The model under review builds one solid part; all positions refer to its coordinate system, in mm. Coordinates: 2 decimals unless noted, no trailing zeros. Order: outer loops, then holes, each group sorted by start corner. A loop starts at its lowest first (then second) coordinate and runs counter-clockwise, first axis right, second up. Notation, with made-up numbers: M 3.5,-2.75 L 18.5,-2.75 A13 ccw 18.5,14.25 Z; hole C 46,-30.75 d8. An arc over 180 degrees is marked long. Answer in a Markdown table with one row per item.
from build123d import *

# Parameters (mm, degrees)
BOSS_EXTRUDE1_DEPTH = 1
SKETCH2_R           = 2.55
CUT_EXTRUDE6_DEPTH  = 2.54
SKETCH3_R           = 1
CUT_EXTRUDE7_DEPTH  = 2.54


with BuildPart() as part:
    # Sketch1 → Boss-Extrude1 (new body)
    with BuildSketch(Plane(origin=(0, 0, 0), x_dir=(1, 0, 0), z_dir=(0, 1, 0))):
        with BuildLine():
            Line((-42.38, -50), (42.38, -50))
            ThreePointArc((42.38, -50), (47.768153673, -47.768153673), (50, -42.38))
            Line((50, -42.38), (50, 42.38))
            ThreePointArc((50, 42.38), (47.768153673, 47.768153673), (42.38, 50))
            Line((42.38, 50), (-42.38, 50))
            ThreePointArc((-42.38, 50), (-47.768153673, 47.768153673), (-50, 42.38))
            Line((-50, 42.38), (-50, -42.38))
            ThreePointArc((-50, -42.38), (-47.768153673, -47.768153673), (-42.38, -50))
        make_face()
    extrude(amount=BOSS_EXTRUDE1_DEPTH)

    # Sketch2 → Cut-Extrude6 (cut)
    with BuildSketch(Plane(origin=(0, 1, 0), x_dir=(1, 0, 0), z_dir=(0, 1, 0))):
        with Locations((0, 40)):
            Circle(SKETCH2_R)
        with Locations((40, 0)):
            Circle(SKETCH2_R)
        with Locations((0, -40)):
            Circle(SKETCH2_R)
        with Locations((-40, 0)):
            Circle(SKETCH2_R)
    extrude(amount=-CUT_EXTRUDE6_DEPTH, mode=Mode.SUBTRACT)

    # Sketch3 → Cut-Extrude7 (cut)
    with BuildSketch(Plane(origin=(0, 1, 0), x_dir=(1, 0, 0), z_dir=(0, 1, 0))):
        with Locations((0, 24)):
            Circle(SKETCH3_R)
        with Locations((24, 0)):
            Circle(SKETCH3_R)
        with Locations((0, -24)):
            Circle(SKETCH3_R)
        with Locations((-24, 0)):
            Circle(SKETCH3_R)
    extrude(amount=-CUT_EXTRUDE7_DEPTH, mode=Mode.SUBTRACT)


solid = part.part
(1) Take a section at B-B (x = -40). Write out the cut boundary in (y, z), then the cut area to 3 significant figures.
Report:
| item | result |
|---|---|
| outline | M 0,-50 L 1,-50 L 1,-2.55 L 0,-2.55 Z; M 0,2.55 L 1,2.55 L 1,50 L 0,50 Z |
| area | 94.9 mm^2 |
(2) Take a section at A-A (z = -40). Write out the cut boundary in (x, y).
Report:
| item | result |
|---|---|
| outline | M -50,0 L -2.55,0 L -2.55,1 L -50,1 Z; M 2.55,0 L 50,0 L 50,1 L 2.55,1 Z |
(3) The part is to be moulded in two halves that separate along X. For faces 1 (the flat face through (-1, 1, -1)), 2 (the cylindrical face through (-42.548, 0.507, -0.112)), 3 (the cylindrical face through (-47.709, 0.493, -47.827)), say which applies: +X half, -X half, draft (parallel to the pull), parting line (faces both ways), or undercut.
Report:
| item | result |
|---|---|
| face 1 | draft |
| face 2 | undercut |
| face 3 | -X half |
(4) To check wall thickness, follow line 1 (Z direction, x = 0, y = 0.2); line 2 (Z direction, x = -24, y = 0.45). State the ranges of each line that lie inside material, in increasing order. Write a range as [from, to].
Report:
| item | result |
|---|---|
| line 1 | [-50, -42.55], [-37.45, -25], [-23, 23], [25, 37.45], [42.55, 50] |
| line 2 | [-50, -1], [1, 50] |
